Source: CAD feature listing. Evaluate the final solid. Frame: model axes, mm. Round coordinates to 2 decimals unless told otherwise and drop trailing zeros. Order: outer loops, then holes, each group sorted by start corner. A loop starts at its lowest first (then second) coordinate and runs counter-clockwise, first axis right, second up. Notation, with made-up numbers: (81.25, 3.25) - (86.25, 3.25) arc R16 cw to (86.25, 23.25) - close; hole circle Ø4 at (-22.5, 73). An arc over 180 degrees is marked (long way). Put each result on its own line as item: value. Start each with the question number.
1) Section B-B on z = 9. Output: boundary loops of the cut face in (x, y), then the cut area to 3 significant figures.
2) Section C-C on z = -143. Output: boundary loops of the cut face in (x, y), then the cut area to 3 significant figures.
3) Line query: probe 1 along Y at (x, z) = (0, -1); probe 2 along Z at (x, y) = (-2, -4.25); probe 3 along Z at (x, y) = (-1.5, -0.5). Output: solid intervals per line, ascending. Write a range as [from, to].
4) Section D-D on x = 0. Output: boundary loops of the cut face in (y, z).
5) Contact query for flat-ended pins moving along their axis: P1, Ø1.5, axis at x = -6.5, z = -52.5, coming from the +Y side; P2, Ø6, axis at y = 0, z = -120, coming from the +X side; P3, Ø10, axis at x = -3, z = -57, coming from the +Y side. Output: stop coordinate, or through.
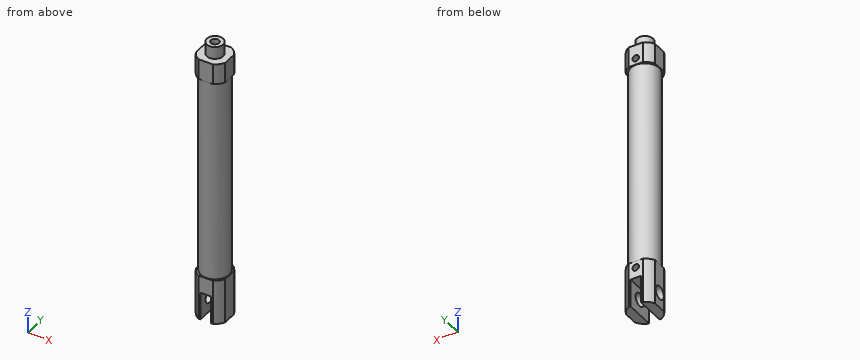
```python
from build123d import *

# Parameters (mm, degrees)
BOSS_EXTRUDE1_DEPTH = 12.5
SKETCH2_R           = 5
BOSS_EXTRUDE2_DEPTH = 7.5
SKETCH3_R           = 8.75
BOSS_EXTRUDE3_DEPTH = 125
BOSS_EXTRUDE4_START = 27.5
BOSS_EXTRUDE4_DEPTH = 27.5
SKETCH7_W           = 6.5
SKETCH7_H           = 18
CUT_EXTRUDE1_DEPTH  = 17
SKETCH8_R           = 4
CUT_EXTRUDE2_DEPTH  = 17
SKETCH9_R           = 2
CUT_EXTRUDE3_DEPTH  = 4
SKETCH10_R          = 2
CUT_EXTRUDE4_DEPTH  = 4
SKETCH11_R          = 2.5
CUT_EXTRUDE5_DEPTH  = 100


with BuildPart() as part:
    # Sketch1 → Boss-Extrude1 (new body)
    with BuildSketch(Plane.XY):
        with BuildLine():
            ThreePointArc((-9, -4.358898944), (-7.071067812, -7.071067812), (-4.358898944, -9))
            Line((-4.358898944, -9), (4.358898944, -9))
            ThreePointArc((4.358898944, -9), (7.071067812, -7.071067812), (9, -4.358898944))
            Line((9, -4.358898944), (9, 4.358898944))
            ThreePointArc((9, 4.358898944), (7.071067812, 7.071067812), (4.358898944, 9))
            Line((4.358898944, 9), (-4.358898944, 9))
            ThreePointArc((-4.358898944, 9), (-7.071067812, 7.071067812), (-9, 4.358898944))
            Line((-9, 4.358898944), (-9, -4.358898944))
        make_face()
    extrude(amount=BOSS_EXTRUDE1_DEPTH)

    # Sketch2 → Boss-Extrude2 (add)
    with BuildSketch(Plane.XY.offset(12.5)):
        Circle(SKETCH2_R)
    extrude(amount=BOSS_EXTRUDE2_DEPTH)

    # Sketch3 → Boss-Extrude3 (add)
    with BuildSketch(Plane(origin=(0, 0, 0), x_dir=(-1, 0, 0), z_dir=(0, 0, -1))):
        with Locations(Location((0, 0, 0), (0, 0, 180))):
            Circle(SKETCH3_R)
    extrude(amount=BOSS_EXTRUDE3_DEPTH)

    # Sketch6 → Boss-Extrude4 (add)
    with BuildSketch(Plane(origin=(0, 0, -125), x_dir=(-1, 0, 0), z_dir=(0, 0, -1)).offset(BOSS_EXTRUDE4_START)):
        with BuildLine():
            Line((-4.358898944, -9), (4.358898944, -9))
            ThreePointArc((4.358898944, -9), (7.071067812, -7.071067812), (9, -4.358898944))
            Line((9, -4.358898944), (9, 4.358898944))
            ThreePointArc((9, 4.358898944), (7.071067812, 7.071067812), (4.358898944, 9))
            Line((4.358898944, 9), (-4.358898944, 9))
            ThreePointArc((-4.358898944, 9), (-7.071067812, 7.071067812), (-9, 4.358898944))
            Line((-9, 4.358898944), (-9, -4.358898944))
            ThreePointArc((-9, -4.358898944), (-7.071067812, -7.071067812), (-4.358898944, -9))
        make_face()
    extrude(amount=-BOSS_EXTRUDE4_DEPTH)

    # Sketch7 → Cut-Extrude1 (cut)
    with BuildSketch(Plane(origin=(0, 0, -152.5), x_dir=(-1, 0, 0), z_dir=(0, 0, -1))):
        Rectangle(SKETCH7_W, SKETCH7_H)
    extrude(amount=-CUT_EXTRUDE1_DEPTH, mode=Mode.SUBTRACT)

    # Sketch8 → Cut-Extrude2 (cut)
    with BuildSketch(Plane.ZY.offset(9)):
        with Locations((-143, 0)):
            Circle(SKETCH8_R)
    extrude(amount=-CUT_EXTRUDE2_DEPTH, mode=Mode.SUBTRACT)

    # Sketch9 → Cut-Extrude3 (cut)
    with BuildSketch(Plane(origin=(0, 9, 0), x_dir=(1, 0, 0), z_dir=(0, 1, 0))):
        with Locations(Location((0, 129, 0), (0, 0, 270))):
            Circle(SKETCH9_R)
    extrude(amount=-CUT_EXTRUDE3_DEPTH, mode=Mode.SUBTRACT)

    # Sketch10 → Cut-Extrude4 (cut)
    with BuildSketch(Plane(origin=(0, 9, 0), x_dir=(1, 0, 0), z_dir=(0, 1, 0))):
        with Locations(Location((0, -4, 0), (0, 0, 180))):
            Circle(SKETCH10_R)
    extrude(amount=-CUT_EXTRUDE4_DEPTH, mode=Mode.SUBTRACT)

    # Sketch11 → Cut-Extrude5 (cut)
    with BuildSketch(Plane.XY.offset(20)):
        Circle(SKETCH11_R)
    extrude(amount=-CUT_EXTRUDE5_DEPTH, mode=Mode.SUBTRACT)


solid = part.part
```
Answer sheet:
1. outline: (-9, -4.36) arc R10 ccw to (-4.36, -9) - (4.36, -9) arc R10 ccw to (9, -4.36) - (9, 4.36) arc R10 ccw to (4.36, 9) - (-4.36, 9) arc R10 ccw to (-9, 4.36) - close; hole circle Ø5 at (0, 0)
1. area: 271 mm^2
2. outline: (-9, -4.36) arc R10 ccw to (-4.36, -9) - (-3.25, -9) - (-3.25, -4) - (-9, -4) - close; (-9, 4) - (-3.25, 4) - (-3.25, 9) - (-4.36, 9) arc R10 ccw to (-9, 4.36) - close; (3.25, -9) - (4.36, -9) arc R10 ccw to (9, -4.36) - (9, 4.36) arc R10 ccw to (4.36, 9) - (3.25, 9) - (3.25, 4) - (8, 4) - (8, -4) - (3.25, -4) - close
2. area: 89.7 mm^2
3. probe 1: [-8.75, -2.5], [2.5, 8.75]
3. probe 2: [-135.5, 20]
3. probe 3: [-135.5, -80]
4. outline: (-9, -135.5) - (9, -135.5) - (9, -131) - (5, -131) - (5, -127) - (9, -127) - (9, -125) - (8.75, -125) - (8.75, 0) - (9, 0) - (9, 2) - (5, 2) - (5, 6) - (9, 6) - (9, 12.5) - (5, 12.5) - (5, 20) - (2.5, 20) - (2.5, -80) - (-2.5, -80) - (-2.5, 20) - (-5, 20) - (-5, 12.5) - (-9, 12.5) - (-9, 0) - (-8.75, 0) - (-8.75, -125) - (-9, -125) - close
5. P1: y = 6.6
5. P2: x = 8.75
5. P3: y = 8.75
